The figure shows three views and two pictorial views of one solid part (mm, origin at its lowest corner). Answer the questions. Give positions to 0.01 mm unless a question says otherwise; leave off trailing zeros. Loops run counter-clockwise (first coordinate to the right, second up) from the corner with the lowest first, then second, coordinate; pieces in that order, holes last. Notation, with made-up numbers: M -32,37.5 L 6,37.5 A24 ccw 6,74.5 Z; hole C 11.5,-20 d1. An arc over 180 degrees is marked long. Write item = value, one per line. Start each with the question number.
1. A flat-ended cylindrical pin translates along its axis: pin 1 Ø3 at (x, y) = (60, 165) entering from -Z. Find the tip coordinate at first contact, or state that the pin passes through.
2. Consider L1, parallel to Y at x = 60, z = 2.1; L2, parallel to Y at x = 180.5, z = 3.4. Determine where each line is inside the solid, lowest interval first. Write a range as [from, to].
3. Section A-A on y = 230.5 is taken. Determine the outline of the cut face in (x, z).
4. Section C-C on x = 133 is taken. Determine the outline of the cut face in (y, z), plus the area to 4 significant figures.
5. Section B-B on z = 2.6 is taken. Determine the outline of the cut face in (x, y), plus the area to 3 significant figures.
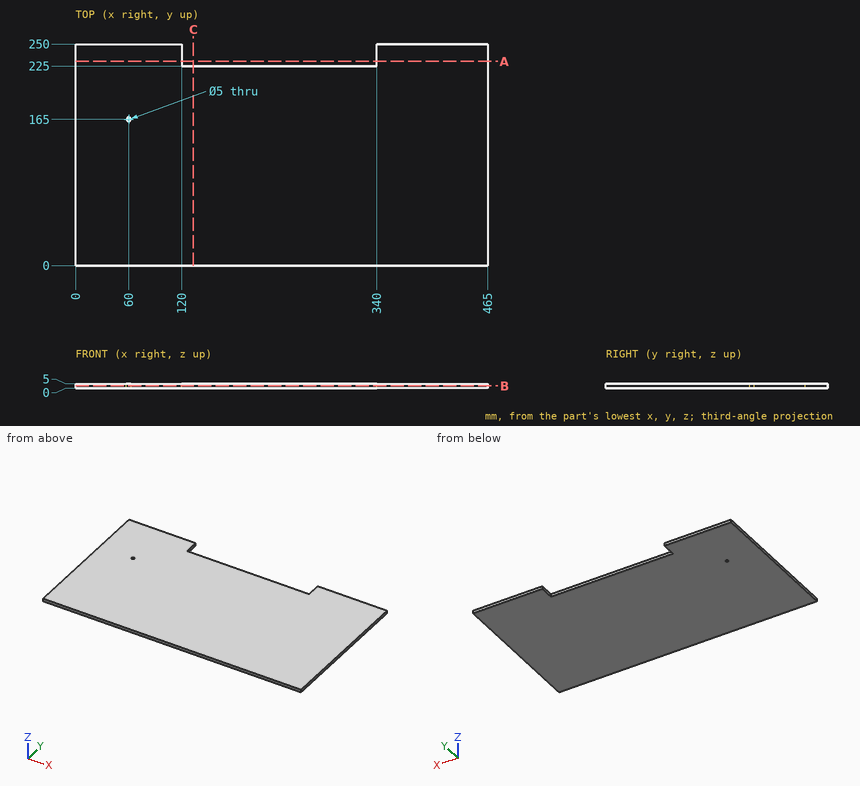
Verdict:
q1.pin_1 = through
q2.L1 = [0, 162.5], [167.5, 250]
q2.L2 = [0, 225]
q3.outline = M 0,0 L 120,0 L 120,5 L 0,5 Z; M 340,0 L 465,0 L 465,5 L 340,5 Z
q4.outline = M 0,0 L 225,0 L 225,5 L 0,5 Z
q4.area = 1,125 mm2
q5.outline = M 0,0 L 465,0 L 465,250 L 340,250 L 340,225 L 120,225 L 120,250 L 0,250 Z; hole C 60,165 d5
q5.area = 111,000 mm2
